Here's how the part is built. I have some questions about the finished solid (model axes, mm). Face numbers are marked on the shaded views. A direction names the side the tool comes from. Coordinates: 2 decimals unless noted, no trailing zeros. Write each loop counter-clockwise with the first axis right and the second up, starting at its lowest first coordinate (ties: lowest second). Pieces come first, ordered by that corner, then holes.
Item 1: If we section it at D-D (y = 6.25): Please give me the cut outline in (x, z), then the cut area to 3 significant figures.
Item 2: I'm going to push flat-ended pins straight in: pin 1 Ø1 at (x, y) = (-0.5, 5.5) entering from +Z; pin 2 Ø2 at (y, z) = (6, -2) entering from -X; pin 3 Ø2.5 at (x, z) = (0, 0) entering from -Y. Where does each tip first touch, or does it pass through?
Item 3: If we section it at A-A (y = 1): Please give me the cut outline in (x, z).
Item 4: We'd pull the mould along X, two halves only. Please class the marked faces 3, 4 and 5: +X half, -X half, draft (parallel to the pull), parting line (faces both ways), or undercut.
Item 5: If we section it at B-B (y = 4): Please give me the cut outline in (x, z), then the cut area to 3 significant figures.
Item 6: For the marked faces 1 and 2, which set-ups out of +Z, -Z, +X, -X, +Y, -Y let a thin tool reach every point of the face, with its end or its side?
Item 7: If I drill on line 1 (Z direction, x = 0, y = 0.4); line 2 (Z direction, x = -0.75, y = 3.25), over which ranges is the centre line in solid material (lowest first)?
Item 8: If we section it at C-C (y = 2.25): Please give me the cut outline in (x, z), then the cut area to 3 significant figures.
from build123d import *

# Parameters (mm, degrees)
FILLET1_R     = 0.127
CHAMFER1_SIZE = 0.762


with BuildPart() as part:
    # Sketch1 → Revolve1 (revolve)
    with BuildSketch(Plane.XY):
        Polygon((0, 6.858), (3.1496, 6.858), (3.1496, 1.778), (2.3749, 1.778), (2.3749, 0), (1.524, 0), (1.524, 1.778), (0, 2.726975536), align=None)
    revolve(axis=Axis((0, 0, 0), (0, 1, 0)))

    # Fillet1
    fillet1_edges = [part.edges().sort_by_distance(p)[0] for p in [
        (-2.3749, 1.778, 0),
    ]]
    fillet(fillet1_edges, radius=FILLET1_R)

    # Chamfer1
    chamfer1_edges = [part.edges().sort_by_distance(p)[0] for p in [
        (-3.1496, 6.858, 0),
    ]]
    chamfer(chamfer1_edges, length=CHAMFER1_SIZE)


solid = part.part
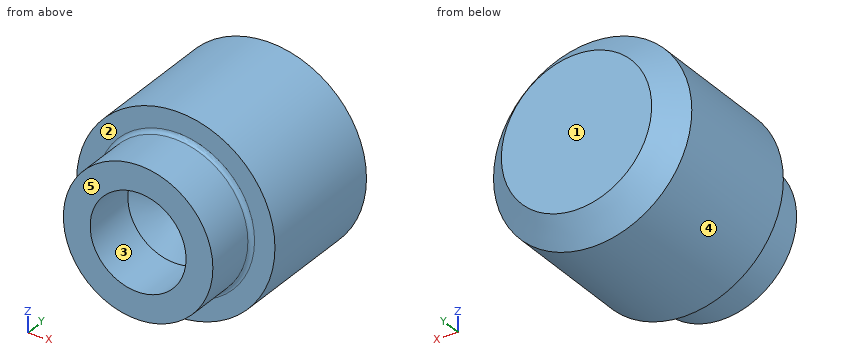
Answer list:
1. outline: circle Ø5.99 at (0, 0)
1. area: 28.2 mm2
2. pin 1: stops at z = 3.15
2. pin 2: stops at x = -2.99
2. pin 3: stops at y = 1.95
3. outline: circle Ø4.75 at (0, 0); hole circle Ø3.05 at (0, 0)
4. face 3: undercut
4. face 4: parting line
4. face 5: draft
5. outline: circle Ø6.3 at (0, 0)
5. area: 31.2 mm2
6. face 1: +Z, -Z, +X, -X, +Y
6. face 2: -Y
7. line 1: z = -2.37 to -1.52, 1.52 to 2.37
7. line 2: z = -3.06 to 3.06
8. outline: circle Ø6.3 at (0, 0); hole circle Ø1.53 at (0, 0)
8. area: 29.3 mm2
